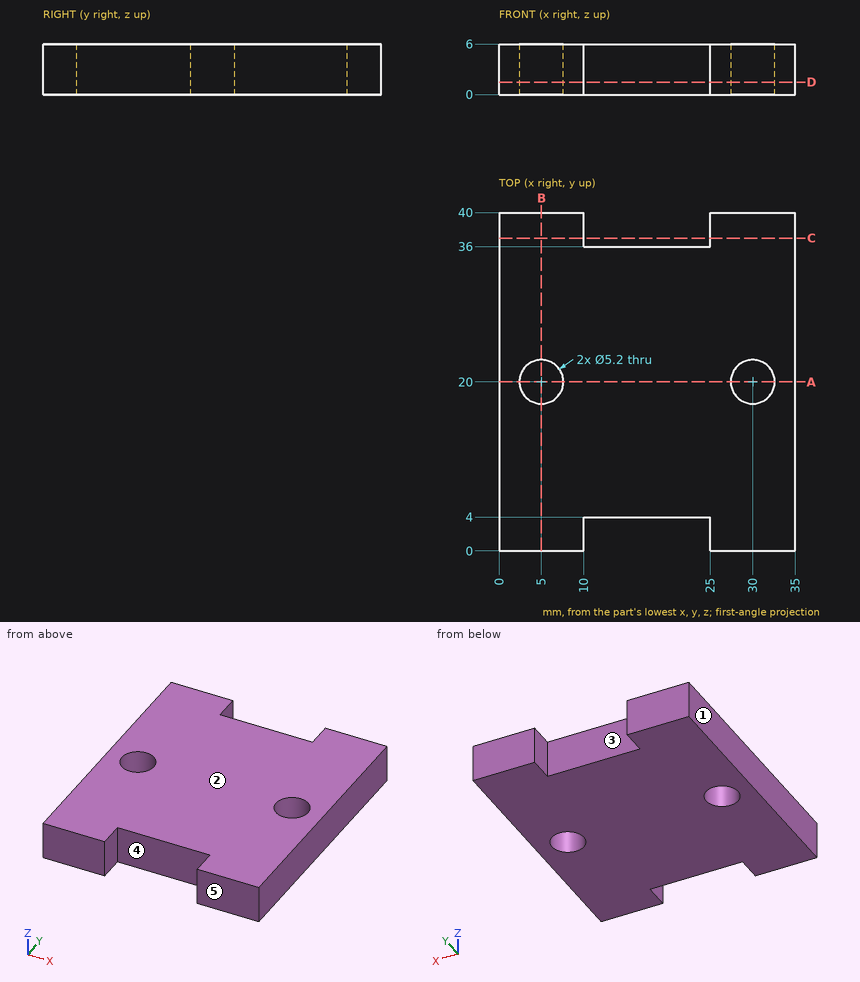
Job drawing, mm, ordinate dimensions from the low corner. One solid piece. A direction names the side the tool comes from. Give positions to 0.01 mm unless a question says otherwise; leave off trailing zeros. Write each loop counter-clockwise with the first axis right and the second up, starting at its lowest first coordinate (ties: lowest second). Pieces come first, ordered by that corner, then holes. Notation, with made-up numbers: M 30.5,57.5 L 65.5,57.5 A29 ccw 65.5,84.5 Z; hole C -3,-26 d6. An arc over 180 degrees is marked long. Put each result on its own line as item: value. Start each with the question number.
(1) Band-saw the part on A-A, the plane y = 20. Write the cut outline in (x, z), and give its area (3 significant figures).
(2) Band-saw the part on B-B, the plane x = 5. Write the cut outline in (y, z).
(3) Band-saw the part on C-C, the plane y = 37. Write the cut outline in (x, z).
(4) Band-saw the part on D-D, the plane z = 1.5. Write the cut outline in (x, y).
(5) Which spindle directions (+Z, -Z, +X, -X, +Y, -Y) get a long thin tool onto all of the face, cutting with end or side? Do the marked faces 4 and 5. Say none if no direction does.
(6) Mould opens along X. For the marked faces 1, 2 and 3 say: +X half, -X half, draft (parallel to the pull), parting line (faces both ways), or undercut.
(7) Probe L1, parallel to X at y = 3.5, z = 2.5; L2, parallel to Y at x = 30, z = 4.45; L3, parallel to Y at x = 14.5, z = 3.15. List the from-to ranges inside material, lowest first.
Response values:
1. outline: M 0,0 L 2.4,0 L 2.4,6 L 0,6 Z; M 7.6,0 L 27.4,0 L 27.4,6 L 7.6,6 Z; M 32.6,0 L 35,0 L 35,6 L 32.6,6 Z
1. area: 148 mm2
2. outline: M 0,0 L 17.4,0 L 17.4,6 L 0,6 Z; M 22.6,0 L 40,0 L 40,6 L 22.6,6 Z
3. outline: M 0,0 L 10,0 L 10,6 L 0,6 Z; M 25,0 L 35,0 L 35,6 L 25,6 Z
4. outline: M 0,0 L 10,0 L 10,4 L 25,4 L 25,0 L 35,0 L 35,40 L 25,40 L 25,36 L 10,36 L 10,40 L 0,40 Z; hole C 5,20 d5.2; hole C 30,20 d5.2
5. face 4: +Z, -Z, -Y
5. face 5: +Z, -Z, +X, -X, -Y
6. face 1: -X half
6. face 2: draft
6. face 3: undercut
7. L1: x = 0 to 10, 25 to 35
7. L2: y = 0 to 17.4, 22.6 to 40
7. L3: y = 4 to 36
